```python
from build123d import *

# Parameters (mm, degrees)
ESBO_O1_R                = 34
ESBO_O1_R_2              = 16
ESBO_O1_R_3              = 3.5
RESSALTO_EXTRUS_O1_DEPTH = 6
CORTE_EXTRUS_O1_START    = -10
CORTE_EXTRUS_O1_DEPTH    = 10


with BuildPart() as part:
    # Esboço1 → Ressalto-extrusão1 (new body)
    with BuildSketch(Plane.XY):
        Circle(ESBO_O1_R)
        Circle(ESBO_O1_R_2, mode=Mode.SUBTRACT)
        with Locations((0, 25.5)):
            Circle(ESBO_O1_R_3, mode=Mode.SUBTRACT)
        with Locations((25.5, 0)):
            Circle(ESBO_O1_R_3, mode=Mode.SUBTRACT)
        with Locations((0, -25.5)):
            Circle(ESBO_O1_R_3, mode=Mode.SUBTRACT)
        with Locations((-25.5, 0)):
            Circle(ESBO_O1_R_3, mode=Mode.SUBTRACT)
    extrude(amount=RESSALTO_EXTRUS_O1_DEPTH)

    # Esboço2 → Corte-extrusão1 (cut)
    with BuildSketch(Plane.XY.offset(6).offset(CORTE_EXTRUS_O1_START)):
        with BuildLine():
            Line((-11.884080362, 31.855433351), (12.162956055, 31.75))
            ThreePointArc((12.162956055, 31.75), (0.149070322, 33.999673205), (-11.884080362, 31.855433351))
        make_face()
    extrude(amount=CORTE_EXTRUS_O1_DEPTH, mode=Mode.SUBTRACT)


solid = part.part
```
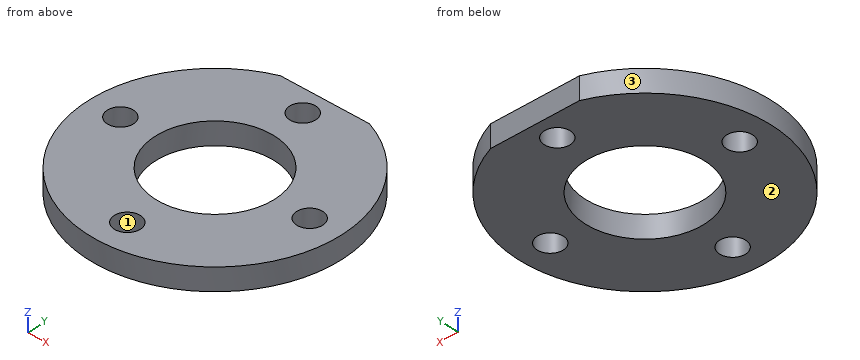
CAD build for the part. Positions are in the model's coordinates, mm. Face numbers are marked on the shaded views. Coordinates: 2 decimals unless noted, no trailing zeros. Order: outer loops, then holes, each group sorted by start corner. A loop starts at its lowest first (then second) coordinate and runs counter-clockwise, first axis right, second up. Notation, with made-up numbers: (-3, -15) -> (14, -15) arc R18 cw to (14, 8) -> close; hole circle Ø10 at (10.5, -20.75). An arc over 180 degrees is marked (long way). Use one line per item in the form item = value. Start each with the question number.
1) Drop flat-ended pins along their axis: pin 1 (9 mm diameter, centred on x = 25.5, y = 0, fed in from +Z); pin 2 (2 mm diameter, centred on x = 26, z = 3, fed in from -Y); pin 3 (1.5 mm diameter, centred on y = -24, z = 3.5, fed in from +X). Give the stop position or say it passes through.
2) Band-saw the part on A-A on x = 25.5. Give the cut face in (y, z).
3) Drill centre lines: L1, parallel to Y at x = 0, z = 4.05; L2, parallel to X at y = -27, z = 5.75; L3, parallel to Y at x = -28.5, z = 3.3. Where is each one in solid material? Low to high. Write a range as [from, to].
4) Band-saw the part on D-D on x = 1.5. Give the cut face in (y, z), then the cut area to 3 significant figures.
5) Pull direction Y, two halves, no side cores. Call the marked faces 1, 2 and 3: +Y half, -Y half, draft (parallel to the pull), parting line (faces both ways), or undercut.
6) Band-saw the part on B-B on y = 0. Give the cut face in (x, z).
Entries:
q1.pin_1 = 6
q1.pin_2 = -23.04
q1.pin_3 = 24.81
q2.outline = (-22.49, 0) -> (-3.5, 0) -> (-3.5, 6) -> (-22.49, 6) -> close; (3.5, 0) -> (22.49, 0) -> (22.49, 6) -> (3.5, 6) -> close
q3.L1 = [-34, -29], [-22, -16], [16, 22], [29, 31.8]
q3.L2 = [-20.66, -3.16], [3.16, 20.66]
q3.L3 = [-18.54, -1.8], [1.8, 18.54]
q4.outline = (-33.97, 0) -> (-28.66, 0) -> (-28.66, 6) -> (-33.97, 6) -> close; (-22.34, 0) -> (-15.93, 0) -> (-15.93, 6) -> (-22.34, 6) -> close; (15.93, 0) -> (22.34, 0) -> (22.34, 6) -> (15.93, 6) -> close; (28.66, 0) -> (31.8, 0) -> (31.8, 6) -> (28.66, 6) -> close
q4.area = 128 mm2
q5.face_1 = undercut
q5.face_2 = draft
q5.face_3 = parting line
q6.outline = (-34, 0) -> (-29, 0) -> (-29, 6) -> (-34, 6) -> close; (-22, 0) -> (-16, 0) -> (-16, 6) -> (-22, 6) -> close; (16, 0) -> (22, 0) -> (22, 6) -> (16, 6) -> close; (29, 0) -> (34, 0) -> (34, 6) -> (29, 6) -> close
